Read the model definition and answer for the solid it produces. Units are mm, in the model's axes. Coordinates: 2 decimals unless noted, no trailing zeros. Write each loop counter-clockwise with the first axis right and the second up, starting at its lowest first coordinate (ties: lowest second). Pieces come first, ordered by that corner, then holes. Notation, with made-up numbers: (69, 24.5) -> (93, 24.5) arc R21 ccw to (93, 29.5) -> close; hole circle Ø5 at (82.25, 44.5). An arc over 180 degrees is marked (long way). Return JSON: item names as keys, results as strings.
from build123d import *

# Parameters (mm, degrees)
ESQUISSE1_W                   = 12
ESQUISSE1_H                   = 1
DIAM_TRE_DU_PER_AGE_5_0_5_1_D = 5
DIAM_TRE_DU_PER_AGE_5_0_5_2_D = 5
R_P_TITION_CIRCULAIRE1_COUNT  = 4


with BuildPart() as part:
    # Esquisse1 → Révolution1 (revolve)
    with BuildSketch(Plane(origin=(0, 0, 0), x_dir=(0, 0, -1), z_dir=(1, 0, 0))):
        with Locations((-36, 0.5)):
            Rectangle(ESQUISSE1_W, ESQUISSE1_H)
    revolve(axis=Axis((0, 0, 0), (0, -1, 0)))

    # Diamètre du perçage Ø5.0 (5)1 (through all)
    with Locations(Plane(origin=(0, 1, 0), x_dir=(1, 0, 0), z_dir=(0, 1, 0))):
        with Locations((0, 37), (0, -37)):
            Hole(DIAM_TRE_DU_PER_AGE_5_0_5_1_D / 2)

    # Diamètre du perçage Ø5.0 (5)2 (through all)
    with Locations(Plane(origin=(0, 1, 0), x_dir=(1, 0, 0), z_dir=(0, 1, 0))):
        with Locations((-26.162950904, 26.162950904)):
            diam_tre_du_per_age_5_0_5_2 = Hole(DIAM_TRE_DU_PER_AGE_5_0_5_2_D / 2)

    # Répétition circulaire1: Diamètre du perçage Ø5.0 (5)2 ×4 about axis
    r_p_tition_circulaire1_axis = Axis((0, 0, 0), (0, 1, 0))
    for i in range(1, R_P_TITION_CIRCULAIRE1_COUNT):
        add(diam_tre_du_per_age_5_0_5_2.rotate(r_p_tition_circulaire1_axis, i * 360 / R_P_TITION_CIRCULAIRE1_COUNT), mode=Mode.SUBTRACT)


solid = part.part
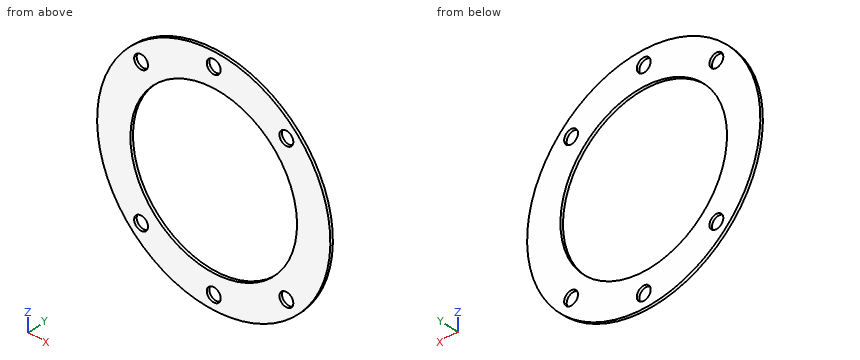
1. The part is cut by section D-D (x = 14). Determine the outline of the cut face in (y, z).
Taken from the geometry:
{"outline": "(0, -39.6) -> (1, -39.6) -> (1, -26.53) -> (0, -26.53) -> close; (0, 26.53) -> (1, 26.53) -> (1, 39.6) -> (0, 39.6) -> close"}
2. The part is cut by section B-B (y = 0.8). Determine the outline of the cut face in (x, z).
Taken from the geometry:
{"outline": "circle Ø84 at (0, 0); hole circle Ø60 at (0, 0); hole circle Ø5 at (-26.16, -26.16); hole circle Ø5 at (-26.16, 26.16); hole circle Ø5 at (0, -37); hole circle Ø5 at (0, 37); hole circle Ø5 at (26.16, -26.16); hole circle Ø5 at (26.16, 26.16)"}
3. The part is cut by section A-A (x = 0). Determine the outline of the cut face in (y, z).
Taken from the geometry:
{"outline": "(0, -42) -> (1, -42) -> (1, -39.5) -> (0, -39.5) -> close; (0, -34.5) -> (1, -34.5) -> (1, -30) -> (0, -30) -> close; (0, 30) -> (1, 30) -> (1, 34.5) -> (0, 34.5) -> close; (0, 39.5) -> (1, 39.5) -> (1, 42) -> (0, 42) -> close"}
4. Consider L1, parallel to Z at x = 0, y = 0.85; L2, parallel to X at y = 0.2, z = 0; L3, parallel to X at y = 0.4, z = 18.5. Determine where each line is inside the solid, lowest interval first.
Taken from the geometry:
{"L1": "z = -42 to -39.5, -34.5 to -30, 30 to 34.5, 39.5 to 42", "L2": "x = -42 to -30, 30 to 42", "L3": "x = -37.71 to -23.62, 23.62 to 37.71"}
5. The part is cut by section C-C (z = -37). Determine the outline of the cut face in (x, y), then the cut area to 3 significant figures.
Taken from the geometry:
{"outline": "(-19.87, 0) -> (-2.5, 0) -> (-2.5, 1) -> (-19.87, 1) -> close; (2.5, 0) -> (19.87, 0) -> (19.87, 1) -> (2.5, 1) -> close", "area": "34.7 mm2"}
